Can you work these out from the model? Positions are in its coordinate system, mm. A direction names the side the tool comes from. Give positions to 0.01 mm unless a question says otherwise; leave off trailing zeros. Loops run counter-clockwise (first coordinate to the right, second up) from the corner with the lowest first, then second, coordinate; pieces in that order, holes last.
from build123d import *

# Parameters (mm, degrees)
F0_W     = 17.5
F0_H     = 5
F1_DEPTH = 2.5
F2_W     = 7.5
F2_H     = 5
F3_DEPTH = 2.5
F4_W     = 2.5
F4_H     = 2.5
F5_DEPTH = 2.5
F6_W     = 2.5
F6_H     = 2.5
F7_DEPTH = 2.5


with BuildPart() as f1:
    # F0 (on Top) → F1 (new body, symmetric)
    with BuildSketch(Plane.XY):
        with Locations((8.75, 2.5)):
            Rectangle(F0_W, F0_H)
        with Locations((-8.75, 2.5)):
            Rectangle(F0_W, F0_H)
    extrude(amount=F1_DEPTH, both=True)

    # F2 (on Top) → F3 (cut)
    with BuildSketch(Plane.XY):
        with Locations((3.75, 2.5)):
            Rectangle(F2_W, F2_H)
        with Locations((-3.75, 2.5)):
            Rectangle(F2_W, F2_H)
    extrude(amount=F3_DEPTH, mode=Mode.SUBTRACT)

    # F4 (on Right) → F5 (cut)
    with BuildSketch(Plane.YZ):
        with Locations((1.25, -1.25)):
            Rectangle(F4_W, F4_H)
    extrude(amount=F5_DEPTH, mode=Mode.SUBTRACT)

    # F6 (on Top) → F7 (join)
    with BuildSketch(Plane.XY):
        with Locations((1.25, 3.75)):
            Rectangle(F6_W, F6_H)
    extrude(amount=F7_DEPTH)


solid = f1.part
(1) Suppose I cut it at D-D on y = 3.8. List the corners of the cut face in (x, z) for me, plus the area to 3 significant figures.
Returned:
outline: (-17.5, -2.5) - (17.5, -2.5) - (17.5, 2.5) - (7.5, 2.5) - (7.5, 0) - (2.5, 0) - (2.5, 2.5) - (0, 2.5) - (0, 0) - (-7.5, 0) - (-7.5, 2.5) - (-17.5, 2.5) - close
area: 144 mm2
(2) Suppose I cut it at C-C on z = -1.05. List the corners of the cut face in (x, y) for me.
Returned:
outline: (-17.5, 0) - (0, 0) - (0, 2.5) - (2.5, 2.5) - (2.5, 0) - (17.5, 0) - (17.5, 5) - (-17.5, 5) - close
(3) Will these pins go through, and if not, where does the flat tip stop? P1, Ø2.5, axis at x = -4, y = 3, coming from the +Z side; P2, Ø0.8, axis at x = 1, z = 0.5, coming from the -Y side.
Returned:
P1: stops at z = 0
P2: stops at y = 2.5
(4) Please list where these lines run through material, in increasing order: probe 1 along X at (y, z) = (3.7, 1.2); probe 2 along X at (y, z) = (1.35, -2.05); probe 3 along X at (y, z) = (1.15, 2.25).
Returned:
probe 1: x = -17.5 to -7.5, 0 to 2.5, 7.5 to 17.5
probe 2: x = -17.5 to 0, 2.5 to 17.5
probe 3: x = -17.5 to -7.5, 7.5 to 17.5
(5) Thinking about a two-plate mould opening in X: for faces 1 (the flat face through (-17.5, 2, 0)), 2 (the flat face through (0, 4, 1)), 3 (the flat face through (0, 5, -1)), which applies, pulls with the +X half, pulls with the -X half, needs draft (parallel to the pull), parting line crosses it, or undercut?
Returned:
face 1: pulls with the -X half
face 2: undercut
face 3: needs draft
(6) Suppose I cut it at A-A on z = 0.4. List the corners of the cut face in (x, y) for me, plus the area to 3 significant figures.
Returned:
outline: (-17.5, 0) - (-7.5, 0) - (-7.5, 5) - (-17.5, 5) - close; (0, 2.5) - (2.5, 2.5) - (2.5, 5) - (0, 5) - close; (7.5, 0) - (17.5, 0) - (17.5, 5) - (7.5, 5) - close
area: 106 mm2
(7) Which directions (+Z, -Z, +X, -X, +Y, -Y) give clear straight access to the entire face, cutting with the end or side of a thin tool? Please do faces 4 (the flat face through (1, 2.5, 0)), 5 (the flat face through (7.5, 2, 1)), 6 (the flat face through (-13, 3, 2.5)).
Returned:
face 4: +Z, -Z, -Y
face 5: +Z, +Y, -Y
face 6: +Z, +X, -X, +Y, -Y
(8) Suppose I cut it at B-B on y = 0.85. List the corners of the cut face in (x, z) for me.
Returned:
outline: (-17.5, -2.5) - (0, -2.5) - (0, 0) - (-7.5, 0) - (-7.5, 2.5) - (-17.5, 2.5) - close; (2.5, -2.5) - (17.5, -2.5) - (17.5, 2.5) - (7.5, 2.5) - (7.5, 0) - (2.5, 0) - close
